from build123d import *

# Parameters (mm, degrees)
SKETCH1_W           = 46
SKETCH1_H           = 10
BOSS_EXTRUDE1_DEPTH = 1.5
FILLET6_R           = 1
BOSS_EXTRUDE2_REACH = 36.377
SKETCH2_W           = 41.6
SKETCH2_H           = 5.6
SKETCH8_W           = 3
SKETCH8_H           = 10
BOSS_EXTRUDE7_DEPTH = 6
FILLET1_R           = 1
FILLET4_R           = 1
SKETCH4_W           = 56
SKETCH4_H           = 25
BOSS_EXTRUDE5_DEPTH = 2
FILLET7_R           = 7
SKETCH6_W           = 12
SKETCH6_H           = 6
CUT_EXTRUDE1_DEPTH  = 41.014028534
CUT_EXTRUDE2_REACH  = 42.014
SKETCH9_W           = 2.5
SKETCH9_H           = 25
CUT_EXTRUDE3_REACH  = 42.014
SKETCH10_W          = 5.4
SKETCH10_H          = 2.2
SKETCH_1_W          = 3
SKETCH_1_H          = 2
CUT_EXTRUDE_1_DEPTH = 39.542995207


with BuildPart() as part:
    # Sketch1 → Boss-Extrude1 (new body)
    with BuildSketch(Plane(origin=(0, 0, 0), x_dir=(1, 0, 0), z_dir=(0, 1, 0))):
        with Locations((0, -20.249999594)):
            Rectangle(SKETCH1_W, SKETCH1_H)
    extrude(amount=BOSS_EXTRUDE1_DEPTH)

    # Fillet6
    fillet6_edges = [part.edges().sort_by_distance(p)[0] for p in [
        (23, 0.75, 25.249999594),
        (-23, 0.75, 25.249999594),
        (-23, 0.75, 15.249999594),
        (23, 0.75, 15.249999594),
    ]]
    fillet(fillet6_edges, radius=FILLET6_R)


with BuildPart() as body_2:
    # Mirror2: mirrored copy
    add(part.part.mirror(Plane.ZX.offset(-1.2)))

    # Sketch2 → Boss-Extrude2 (add, up to next)
    with BuildSketch(Plane(origin=(0, 0, 0), x_dir=(1, 0, 0), z_dir=(0, 1, 0)), mode=Mode.PRIVATE) as boss_extrude2_sk1:
        with Locations((0, -20.249999594)):
            Rectangle(SKETCH2_W, SKETCH2_H)
    boss_extrude2_tool1 = extrude(boss_extrude2_sk1.sketch, amount=-BOSS_EXTRUDE2_REACH, mode=Mode.PRIVATE) - body_2.part

    add(part.part)  # Boss-Extrude2 merges part
    add(boss_extrude2_tool1.solids().sort_by_distance((0, 0, 20.25))[0])

    # Sketch8 → Boss-Extrude7 (add)
    with BuildSketch(Plane(origin=(0, 1.5, 0), x_dir=(1, 0, 0), z_dir=(0, 1, 0))):
        with Locations((6, -20.249999594)):
            Rectangle(SKETCH8_W, SKETCH8_H)
    extrude(amount=BOSS_EXTRUDE7_DEPTH)

    # Mirror4: body 2 across plane


with BuildPart() as body_2_1:
    add(body_2.part)
    add(body_2.part.mirror(Plane(origin=(0, 0, 0), x_dir=(0, 0, 1), z_dir=(1, 0, 0))))

    # Fillet1
    fillet1_edges = [body_2_1.edges().sort_by_distance(p)[0] for p in [
        (-20.8, -1.2, 17.449999594),
        (20.8, -1.2, 17.449999594),
        (-20.8, -1.2, 23.049999594),
        (20.8, -1.2, 23.049999594),
    ]]
    fillet(fillet1_edges, radius=FILLET1_R)

    # Fillet4
    fillet4_edges = [body_2_1.edges().sort_by_distance(p)[0] for p in [
        (-7.5, 4.5, 15.249999594),
        (7.5, 4.5, 25.249999594),
        (7.5, 4.5, 15.249999594),
        (-7.5, 4.5, 25.249999594),
    ]]
    fillet(fillet4_edges, radius=FILLET4_R)

    # Sketch4 → Boss-Extrude5 (add)
    with BuildSketch(Plane(origin=(0, 7.5, 0), x_dir=(1, 0, 0), z_dir=(0, 1, 0))):
        with Locations((0, -12.749999594)):
            Rectangle(SKETCH4_W, SKETCH4_H)
    extrude(amount=BOSS_EXTRUDE5_DEPTH)

    # Fillet7
    fillet7_edges = [body_2_1.edges().sort_by_distance(p)[0] for p in [
        (-28, 8.5, 0.249999594),
        (-28, 8.5, 25.249999594),
        (28, 8.5, 25.249999594),
        (28, 8.5, 0.249999594),
    ]]
    fillet(fillet7_edges, radius=FILLET7_R)

    # Sketch6 → Cut-Extrude1 (cut, through all)
    with BuildSketch(Plane(origin=(0, 9.5, 0), x_dir=(1, 0, 0), z_dir=(0, 1, 0))):
        with Locations((0, -3.249999594)):
            Rectangle(SKETCH6_W, SKETCH6_H)
    extrude(amount=-CUT_EXTRUDE1_DEPTH, mode=Mode.SUBTRACT)

    # Sketch9 → Cut-Extrude2 (cut, up to next)
    with BuildSketch(Plane(origin=(0, 9.5, 0), x_dir=(1, 0, 0), z_dir=(0, 1, 0)), mode=Mode.PRIVATE) as cut_extrude2_sk1:
        with Locations((-26.75, -5.449999594)):
            Rectangle(SKETCH9_W, SKETCH9_H)
    cut_extrude2_tool1 = extrude(cut_extrude2_sk1.sketch, amount=-CUT_EXTRUDE2_REACH, mode=Mode.PRIVATE) & body_2_1.part
    # Sketch9 → Cut-Extrude2 (cut, up to next)
    with BuildSketch(Plane(origin=(0, 9.5, 0), x_dir=(1, 0, 0), z_dir=(0, 1, 0)), mode=Mode.PRIVATE) as cut_extrude2_sk2:
        with Locations((26.75, -5.449999594)):
            Rectangle(SKETCH9_W, SKETCH9_H)
    cut_extrude2_tool2 = extrude(cut_extrude2_sk2.sketch, amount=-CUT_EXTRUDE2_REACH, mode=Mode.PRIVATE) & body_2_1.part
    add(cut_extrude2_tool1.solids().sort_by_distance((-26.75, 9.5, 5.45))[0], mode=Mode.SUBTRACT)
    add(cut_extrude2_tool2.solids().sort_by_distance((26.75, 9.5, 5.45))[0], mode=Mode.SUBTRACT)

    # Sketch10 → Cut-Extrude3 (cut, up to next)
    with BuildSketch(Plane(origin=(0, 9.5, 0), x_dir=(1, 0, 0), z_dir=(0, 1, 0)), mode=Mode.PRIVATE) as cut_extrude3_sk1:
        with Locations((14.5, -1.349999594)):
            Rectangle(SKETCH10_W, SKETCH10_H)
    cut_extrude3_tool1 = extrude(cut_extrude3_sk1.sketch, amount=-CUT_EXTRUDE3_REACH, mode=Mode.PRIVATE) & body_2_1.part
    # Sketch10 → Cut-Extrude3 (cut, up to next)
    with BuildSketch(Plane(origin=(0, 9.5, 0), x_dir=(1, 0, 0), z_dir=(0, 1, 0)), mode=Mode.PRIVATE) as cut_extrude3_sk2:
        with Locations((-14.5, -1.349999594)):
            Rectangle(SKETCH10_W, SKETCH10_H)
    cut_extrude3_tool2 = extrude(cut_extrude3_sk2.sketch, amount=-CUT_EXTRUDE3_REACH, mode=Mode.PRIVATE) & body_2_1.part
    add(cut_extrude3_tool1.solids().sort_by_distance((14.5, 9.5, 1.35))[0], mode=Mode.SUBTRACT)
    add(cut_extrude3_tool2.solids().sort_by_distance((-14.5, 9.5, 1.35))[0], mode=Mode.SUBTRACT)

    # Эскиз1 → Вырез-Вытянуть1 (cut, through all)
    with BuildSketch(Plane.XZ.offset(-1.5)):
        with Locations((0, 24.249999594)):
            Rectangle(SKETCH_1_W, SKETCH_1_H)
    extrude(amount=CUT_EXTRUDE_1_DEPTH, mode=Mode.SUBTRACT)


solid = body_2_1.part
Here's how the part is built. I have some questions about the finished solid (model axes, mm). A direction names the side the tool comes from. Give positions to 0.01 mm unless a question says otherwise; leave off trailing zeros. Loops run counter-clockwise (first coordinate to the right, second up) from the corner with the lowest first, then second, coordinate; pieces in that order, holes last. Notation, with made-up numbers: (-5.75, 40.25) -> (3.25, 40.25) arc R21 cw to (3.25, 50.25) -> close; hole circle Ø7 at (-24.5, 58.25). An arc over 180 degrees is marked (long way). Answer as a JSON object with one key per item and string values. Group by question number.
Item 1: Will these pins go through, and if not, where does the flat tip stop? pin 1 (4 mm diameter, centred on x = 7, y = 5, fed in from -Z); pin 2 (2 mm diameter, centred on x = -26, y = 8.5, fed in from -Z); pin 3 (1.6 mm diameter, centred on y = 8.5, z = 4.5, fed in from +X).
Item 2: Imagine slicing it at D-D on y = -3. Write out the boundary of the cut face in (x, z), then the cut area to 3 significant figures.
Item 3: Imagine slicing it at A-A on y = 4.75. Write out the boundary of the cut face in (x, z).
Item 4: Imagine slicing it at B-B on x = 16. Write out the boundary of the cut face in (y, z), then the cut area to 3 significant figures.
Item 5: Thinking about a two-plate mould opening in Y: for faces 4 (the flat face through (20.8, -1, 20)), 5 (the flat face through (25.5, 9, 10)), which applies, pulls with the +Y half, pulls with the -Y half, needs draft (parallel to the pull), parting line crosses it, or undercut?
Item 6: On a 3-axis mill with a long thin cutter (end or side, diameter ignored), from which of +Z, -Z, +X, -X, +Y, -Y can I reach the whole of each face in a straight line? I mean faces 1 (the cylindrical face through (-20.499, -1.217, 17.735)), 2 (the flat face through (0, -1, 17.45)), 3 (the cylindrical face through (22.699, 0.76, 24.965)). Say none if no direction works.
Item 7: I need wall thicknesses on L1, parallel to Y at x = 16.5, z = 23.5; L2, parallel to Y at x = -15, z = 18.25; L3, parallel to X at y = -2.75, z = 23. Which ranges of each line are inside material? Lowest first, please.
Item 8: Imagine slicing it at C-C on z = 4.25. Write out the boundary of the cut face in (x, y), then the cut area to 3 significant figures.
Answer list:
{
 "1": {"pin 1": "stops at z = 15.25", "pin 2": "stops at z = 1.51", "pin 3": "stops at x = 25.5"},
 "2": {"outline": "(-23, 16.25) arc R1 ccw to (-22, 15.25) -> (22, 15.25) arc R1 ccw to (23, 16.25) -> (23, 24.25) arc R1 ccw to (22, 25.25) -> (1.5, 25.25) -> (1.5, 23.25) -> (-1.5, 23.25) -> (-1.5, 25.25) -> (-22, 25.25) arc R1 ccw to (-23, 24.25) -> close", "area": "453 mm2"},
 "3": {"outline": "(-7.5, 16.25) arc R1 ccw to (-6.5, 15.25) -> (-4.5, 15.25) -> (-4.5, 25.25) -> (-6.5, 25.25) arc R1 ccw to (-7.5, 24.25) -> close; (4.5, 15.25) -> (6.5, 15.25) arc R1 ccw to (7.5, 16.25) -> (7.5, 24.25) arc R1 ccw to (6.5, 25.25) -> (4.5, 25.25) -> close"},
 "4": {"outline": "(-3.9, 15.25) -> (-2.4, 15.25) -> (-2.4, 17.45) -> (0, 17.45) -> (0, 15.25) -> (1.5, 15.25) -> (1.5, 25.25) -> (0, 25.25) -> (0, 23.05) -> (-2.4, 23.05) -> (-2.4, 25.25) -> (-3.9, 25.25) -> close; (7.5, 2.45) -> (9.5, 2.45) -> (9.5, 25.25) -> (7.5, 25.25) -> close", "area": "89.0 mm2"},
 "5": {"face 4": "undercut", "face 5": "needs draft"},
 "6": {"face 1": "-Z, -X", "face 2": "-Z, +X, -X", "face 3": "+Z, +X, -Y"},
 "7": {"L1": "y = -3.9 to -2.4, 0 to 1.5, 7.5 to 9.5", "L2": "y = -3.9 to 1.5, 7.5 to 9.5", "L3": "x = -23 to 23"},
 "8": {"outline": "(-25.5, 7.5) -> (-6, 7.5) -> (-6, 9.5) -> (-25.5, 9.5) -> close; (6, 7.5) -> (25.5, 7.5) -> (25.5, 9.5) -> (6, 9.5) -> close", "area": "78.0 mm2"}
}
